```python
from build123d import *

# Parameters (mm, degrees)
F1_DEPTH    = 0.5
F2_R        = 1.75
F3_DEPTH    = 5.6
F4_T1_DEPTH = 21.3501190522
F4_T3_DEPTH = 21.4204938405


# Not quite as in the source:
# - a fillet or chamfer that OpenCascade refuses, or shapes differently, is made with other operations: its cross-section is extruded or revolved along the edge and cut away or added


with BuildPart() as f1:
    # F0 (on Top) → F1 (new body, symmetric)
    with BuildSketch(Plane.XY):
        Polygon((12.7, -7.62), (12.7, 7.62), (9.1240987852, 7.62), (9.1240987852, 5.62), (4.1240987852, 5.62), (4.1240987852, 7.62), (-4.0011659991, 7.62), (-4.0011659991, 5.62), (-9.0011659991, 5.62), (-9.0011659991, 7.62), (-12.7, 7.62), (-12.7, -7.62), (-9.0011659991, -7.62), (-9.0011659991, -5.62), (-4.0011659991, -5.62), (-4.0011659991, -7.62), (4.1240987852, -7.62), (4.1240987852, -5.62), (9.1240987852, -5.62), (9.1240987852, -7.62), align=None)
    extrude(amount=F1_DEPTH, both=True)

    # F2 (on Front) → F3 (join, symmetric)
    with BuildSketch(Plane.XZ):
        with BuildLine():
            Line((-2.2954130392, -0.004001643), (-2.2954130392, 0.7802180896))
            ThreePointArc((-2.2954130392, 0.7802180896), (-6.588071973, 4.326288954), (-10.8247913043, 0.7135685656))
            Line((-10.8247913043, 0.7135685656), (-10.8191841297, -0.004001643))
            Line((-10.8191841297, -0.004001643), (-6.5542345937, -0.004001643))
            Line((-6.5542345937, -0.004001643), (-2.2954130392, -0.004001643))
        make_face()
        with Locations((-6.5542345937, 2.2683413699)):
            Circle(F2_R, mode=Mode.SUBTRACT)
        with BuildLine():
            Line((10.8930142596, 0), (10.861883565, 0.7857921351))
            ThreePointArc((10.861883565, 0.7857921351), (6.5823484291, 4.3273176658), (2.3028132932, 0.7857921351))
            Line((2.3028132932, 0.7857921351), (2.3028132932, 0))
            Line((2.3028132932, 0), (10.8930142596, 0))
        make_face()
        with Locations((6.5823484291, 2.2683413699)):
            Circle(F2_R, mode=Mode.SUBTRACT)
    extrude(amount=F3_DEPTH, both=True)

    # F4: fillet of radius 4.104163056 on 4 edges, made by hand

    # F4_s2 → F4_t1 (cut)
    with BuildSketch(Plane.XY.offset(-10.6750595261)):
        with BuildLine():
            ThreePointArc((9.1240987852, -7.62), (11.6790355366, -6.2588580306), (12.7, -3.5499761896))
            Line((12.7, -3.5499761896), (12.7, -7.62))
            Line((12.7, -7.62), (9.1240987852, -7.62))
        make_face()
        with BuildLine():
            ThreePointArc((12.7, 3.5499761896), (11.6790355366, 6.2588580306), (9.1240987852, 7.62))
            Line((9.1240987852, 7.62), (12.7, 7.62))
            Line((12.7, 7.62), (12.7, 3.5499761896))
        make_face()
    extrude(amount=F4_T1_DEPTH, mode=Mode.SUBTRACT)

    # F4_s4 → F4_t3 (cut)
    with BuildSketch(Plane.XY.offset(-10.7102469202)):
        with BuildLine():
            ThreePointArc((-9.0011659991, 7.62), (-11.6378503335, 6.2909527611), (-12.7, 3.5359012319))
            Line((-12.7, 3.5359012319), (-12.7, 7.62))
            Line((-12.7, 7.62), (-9.0011659991, 7.62))
        make_face()
        with BuildLine():
            ThreePointArc((-12.7, -3.5359012319), (-11.6378503335, -6.2909527611), (-9.0011659991, -7.62))
            Line((-9.0011659991, -7.62), (-12.7, -7.62))
            Line((-12.7, -7.62), (-12.7, -3.5359012319))
        make_face()
    extrude(amount=F4_T3_DEPTH, mode=Mode.SUBTRACT)


solid = f1.part
```
Design review of the part built by this model. Coordinates are the model's own, in mm. A direction names the side the tool comes from. Give positions to 0.01 mm unless a question says otherwise; leave off trailing zeros. Write each loop counter-clockwise with the first axis right and the second up, starting at its lowest first coordinate (ties: lowest second). Pieces come first, ordered by that corner, then holes. Notation, with made-up numbers: (-25.75, 17) - (28.25, 17) arc R31 ccw to (28.25, 56) - close; hole circle Ø10 at (15, -20). An arc over 180 degrees is marked (long way). Return JSON: item names as keys, results as strings. Group by question number.
(1) Machinability: for faces 5 (the cylindrical face through (-6.503, 0.078, 4.326)), 6 (the flat face through (8.4, 5.6, 1.6)), 7 (the flat face through (-4.001, -7, 0)), 8 (the flat face through (-4.001, 7, 0)), which of the approach directions +Z, -Z, +X, -X, +Y, -Y give a long, thin tool a straight path to every point of the face, cutting with its end or side? Answer none if there is none.
(2) To check wall thickness, follow probe 1 along X at (y, z) = (-4.25, 1.8); probe 2 along X at (y, z) = (0.5, 1.25); probe 3 along Z at (x, y) = (0.5, 5.25). State the ranges of each line that lie inside material, in increasing order.
(3) We need section B-B, the plane z = 3.45. Give the boundary of the cut face in (x, y).
(4) We need section C-C, the plane y = -5. Give the boundary of the cut face in (x, z), then the cut area to 3 significant figures.
(5) We need section D-D, the plane z = 0.15. Give the boundary of the cut face in (x, y), then the cut area to 3 significant figures.
(6) Insertion check: pin 1 (2 mm diameter, centred on x = 4, y = 2, fed in from +Z); pin 2 (0.5 mm diameter, centred on y = 7, z = 0, fed in from +X); pin 3 (1.1 mm diameter, centred on x = 6, z = 0, fed in from -Y). Each pin has a flat end and moves straight along its axis. Give the tip position at first contact, or say it passes through.
(7) Mouldability with a two-part tool opening along X and no side actions: class faces 1 (the flat face through (12.7, 0, 0)), 2 (the flat face through (7, -5.62, 0)), 3 (the flat face through (0, -7.62, 0)), 4 (the cylindrical face through (-11.61, 6.32, -0.01)) as +X half, -X half, draft (parallel to the pull), parting line (faces both ways), or undercut.
Reported:
{
 "1": {"face 5": "+Z, +Y, -Y", "face 6": "+Z, +X, -X, +Y", "face 7": "+Z, -Z, -Y", "face 8": "+Z, -Z, +Y"},
 "2": {"probe 1": "x = -10.49 to -8.24, -4.87 to -2.62, 2.63 to 4.9, 8.27 to 10.54", "probe 2": "x = -10.7 to -7.98, -5.13 to -2.41, 2.42 to 5.16, 8.01 to 10.75", "probe 3": "z = -0.5 to 0.5"},
 "3": {"outline": "(-9.17, -5.6) - (-7.85, -5.6) - (-7.85, 5.6) - (-9.17, 5.6) - close; (-5.26, -5.6) - (-3.94, -5.6) - (-3.94, 5.6) - (-5.26, 5.6) - close; (3.96, -5.6) - (5.29, -5.6) - (5.29, 5.6) - (3.96, 5.6) - close; (7.87, -5.6) - (9.2, -5.6) - (9.2, 5.6) - (7.87, 5.6) - close"},
 "4": {"outline": "(-12.43, -0.5) - (12.44, -0.5) - (12.44, 0.5) - (10.87, 0.5) - (10.86, 0.79) arc R4.36 ccw to (2.3, 0.79) - (2.3, 0.5) - (-2.3, 0.5) - (-2.3, 0.78) arc R4.33 ccw to (-10.82, 0.71) - (-10.82, 0.5) - (-12.43, 0.5) - close; hole circle Ø3.5 at (-6.55, 2.27); hole circle Ø3.5 at (6.58, 2.27)", "area": "55.9 mm2"},
 "5": {"outline": "(-12.7, -3.54) arc R4.1 ccw to (-9, -7.62) - (-9, -5.62) - (-4, -5.62) - (-4, -7.62) - (4.12, -7.62) - (4.12, -5.62) - (9.12, -5.62) - (9.12, -7.62) arc R4.1 ccw to (12.7, -3.55) - (12.7, 3.55) arc R4.1 ccw to (9.12, 7.62) - (9.12, 5.62) - (4.12, 5.62) - (4.12, 7.62) - (-4, 7.62) - (-4, 5.62) - (-9, 5.62) - (-9, 7.62) arc R4.1 ccw to (-12.7, 3.54) - close", "area": "333 mm2"},
 "6": {"pin 1": "stops at z = 4.03", "pin 2": "stops at x = 11.17", "pin 3": "stops at y = -5.62"},
 "7": {"face 1": "+X half", "face 2": "undercut", "face 3": "draft", "face 4": "-X half"}
}
